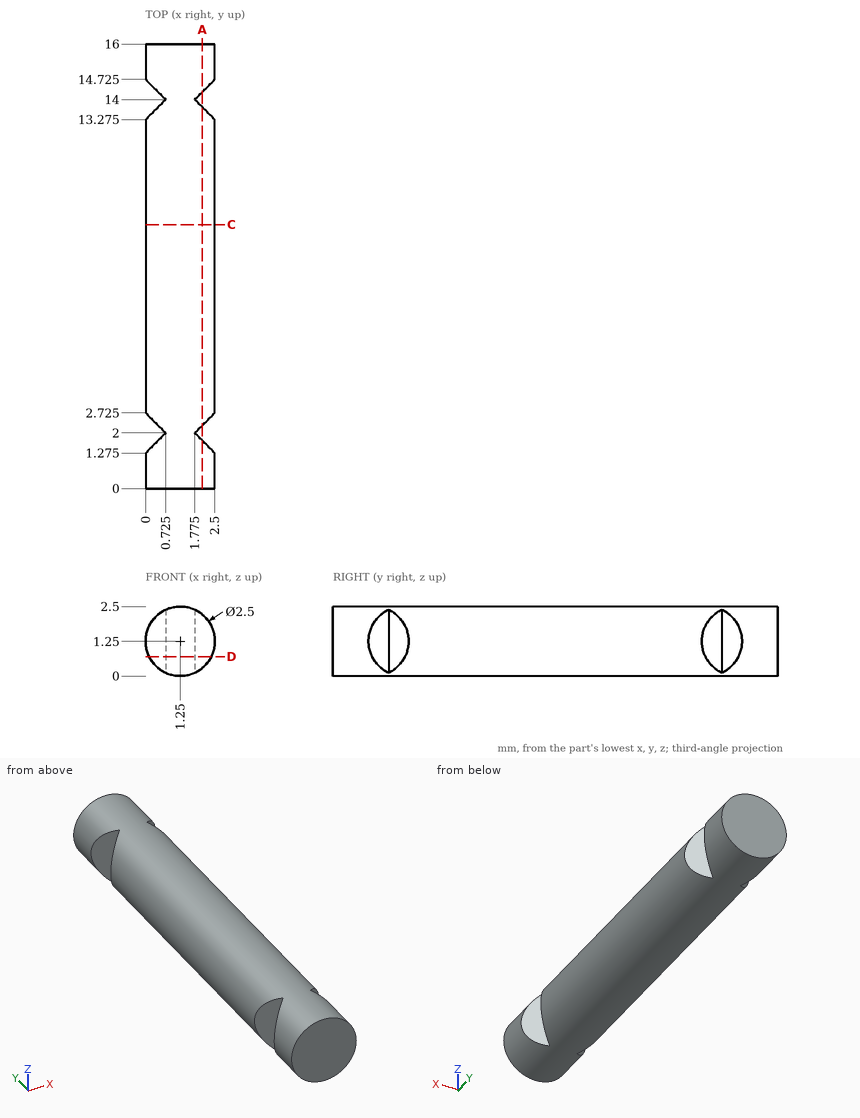
Verification items for this drawing (mm, ordinates from the low corner). Round coordinates to 2 decimals unless told otherwise and drop trailing zeros. Order: outer loops, then holes, each group sorted by start corner. A loop starts at its lowest first (then second) coordinate and runs counter-clockwise, first axis right, second up. Notation, with made-up numbers: (20, 86) - (66, 86) arc R25 ccw to (66, 100) - close; hole circle Ø10 at (-18.5, -33.75). An arc over 180 degrees is marked (long way). Use CSV: the item, a comma, the result in double quotes.
(1) Section check D-D on z = 0.7. Record the boundary of the cut face in (x, y) (1 decimal), and give its area (3 significant figures).
Entries:
outline,"(0.1, 0) - (2.4, 0) - (2.4, 1.4) - (1.8, 2) - (2.4, 2.6) - (2.4, 13.4) - (1.8, 14) - (2.4, 14.6) - (2.4, 16) - (0.1, 16) - (0.1, 14.6) - (0.7, 14) - (0.1, 13.4) - (0.1, 2.6) - (0.7, 2) - (0.1, 1.4) - close"
area,"34.5 mm^2"
(2) Section check A-A on x = 2.05. Record the boundary of the cut face in (y, z) (1 decimal), and give its area (3 significant figures).
Entries:
outline,"(0, 0.3) - (1.7, 0.3) - (1.7, 2.2) - (0, 2.2) - close; (2.3, 0.3) - (13.7, 0.3) - (13.7, 2.2) - (2.3, 2.2) - close; (14.3, 0.3) - (16, 0.3) - (16, 2.2) - (14.3, 2.2) - close"
area,"28.6 mm^2"
(3) Section check C-C on y = 9.5. Record the boundary of the cut face in (x, z).
Entries:
outline,"circle Ø2.5 at (1.25, 1.25)"
(4) Thickness scan on probe 1 along Y at (x, z) = (0.45, 0.4) (1 decimal); probe 2 along Y at (x, z) = (1.9, 0.45) (1 decimal); probe 3 along Z at (x, y) = (1.2, 9). Record the ranges inside material, lowest first. Write a range as from..to.
Entries:
probe 1,"0..1.7, 2.3..13.7, 14.3..16"
probe 2,"0..1.9, 2.1..13.9, 14.1..16"
probe 3,"0..2.5"
